Here's the drawing with two shaded views (mm, measured from the low corner). I have some questions. A direction names the side the tool comes from. Coordinates: 2 decimals unless noted, no trailing zeros. Order: outer loops, then holes, each group sorted by start corner. A loop starts at its lowest first (then second) coordinate and runs counter-clockwise, first axis right, second up. Notation, with made-up numbers: (-31, -37) - (-24, -37) arc R24 cw to (-24, -16) - close; hole circle Ø1 at (32.5, 28). An arc over 180 degrees is marked (long way). Answer as CSV lines item,"result". Start each with the question number.
1. For pin 1 (5.5 mm diameter, centred on x = 18.5, z = 48, fed in from -Y); pin 2 (0.6 mm diameter, centred on y = 8.5, z = 1, fed in from -X) (3 decimals); pin 3 (3.5 mm diameter, centred on y = 10.5, z = 47.5, fed in from +X) (3 decimals); pin 4 (8 mm diameter, centred on y = 13, z = 21.5, fed in from -X), each with a flat end and sliding along its axis, tell me the tip position at first contact or that it passes through.
2. Thinking about a two-plate mould opening in Z: for the marked faces 1, 2 and 3, which applies, released by +Z, released by -Z, zero draft, split by the parting line, or undercut?
3. I want a section at B-B, the plane y = 13.25. List the corners of the cut face in (x, z) for me (3 decimals).
4. I want a section at C-C, the plane z = 17. List the corners of the cut face in (x, y) for me.
5. I want a section at A-A, the plane z = 45.63. List the corners of the cut face in (x, y) for me (3 decimals).
6. For the marked faces 4, 5, 6 and 7, which set-ups out of +Z, -Z, +X, -X, +Y, -Y let a thin tool reach every point of the face, with its end or its side?
7. I need wall thicknesses on probe 1 along X at (y, z) = (3.15, 45.63) (3 decimals); probe 2 along Z at (x, y) = (13.5, 9); probe 3 along Z at (x, y) = (7, 2.5). Which ranges of each line are inside material? Lowest first, please.
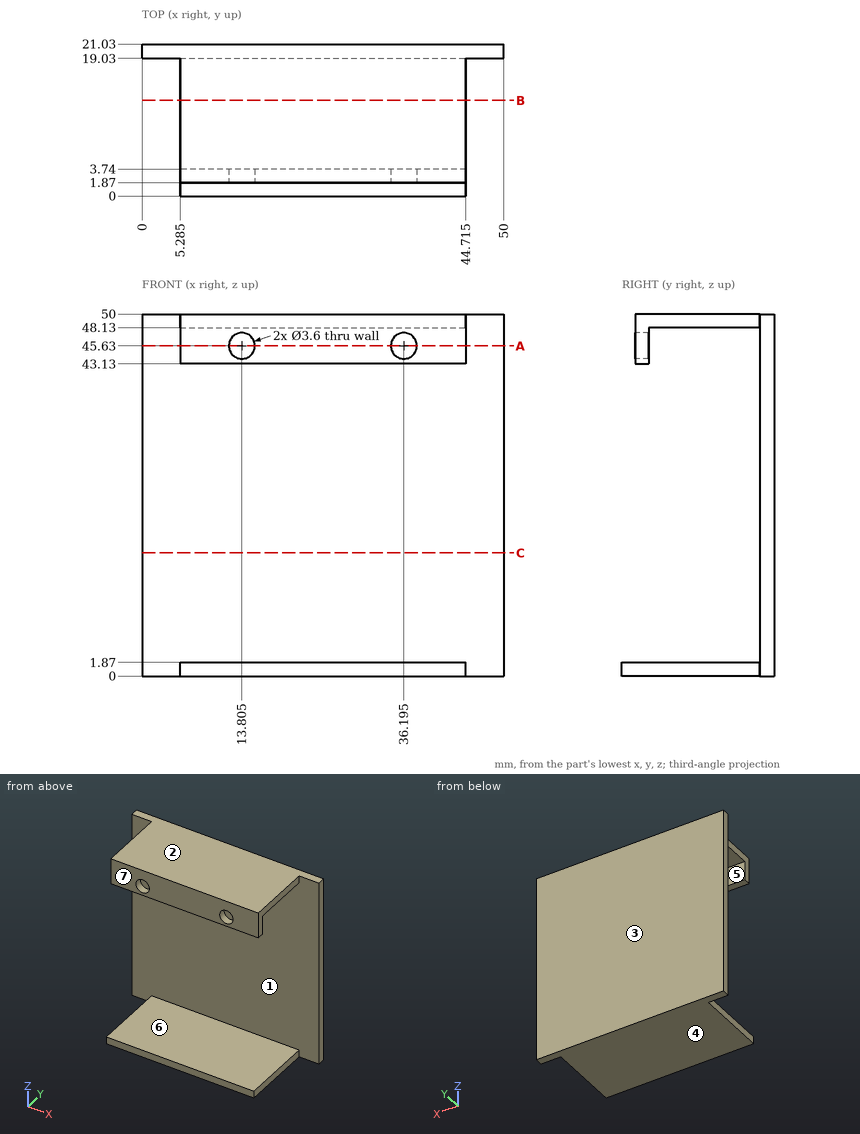
Solved:
1,pin 1,"stops at y = 1.87"
1,pin 2,"stops at x = 5.285"
1,pin 3,"stops at x = 44.715"
1,pin 4,"passes through"
2,face 1,"undercut"
2,face 2,"released by +Z"
2,face 3,"zero draft"
3,outline,"(5.285, 0) - (44.715, 0) - (44.715, 1.87) - (5.285, 1.87) - close; (5.285, 48.13) - (44.715, 48.13) - (44.715, 50) - (5.285, 50) - close"
4,outline,"(0, 19.03) - (50, 19.03) - (50, 21.03) - (0, 21.03) - close"
5,outline,"(0, 19.03) - (50, 19.03) - (50, 21.03) - (0, 21.03) - close; (5.285, 1.87) - (12.005, 1.87) - (12.005, 3.74) - (5.285, 3.74) - close; (15.605, 1.87) - (34.395, 1.87) - (34.395, 3.74) - (15.605, 3.74) - close; (37.995, 1.87) - (44.715, 1.87) - (44.715, 3.74) - (37.995, 3.74) - close"
6,face 4,"-Z, +X, -X, +Y, -Y"
6,face 5,"+X, -X"
6,face 6,"+X, -X, -Y"
6,face 7,"+Z, +X, -X, -Y"
7,probe 1,"x = 5.285 to 12.005, 15.605 to 34.395, 37.995 to 44.715"
7,probe 2,"z = 0 to 1.87, 48.13 to 50"
7,probe 3,"z = 0 to 1.87, 43.13 to 50"
